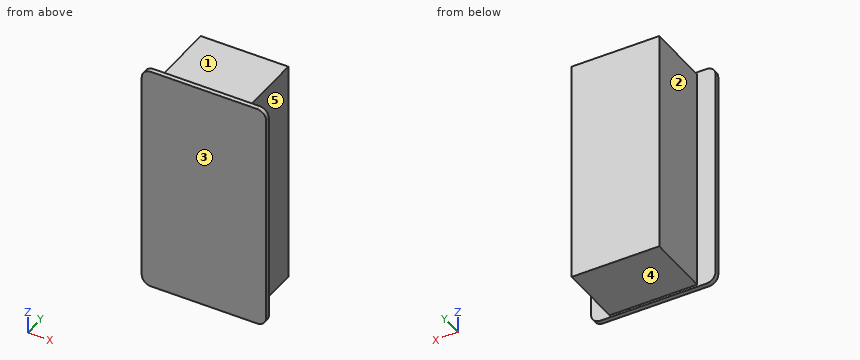
Autodesk Inventor part; units mm, degrees
ref_plane "YZ Plane" through (0, 0, 0) normal (1, 0, 0) x (0, 1, 0)
ref_plane "XZ Plane" through (0, 0, 0) normal (0, 1, 0) x (-1, 0, 0)
ref_plane "XY Plane" through (0, 0, 0) normal (0, 0, 1) x (1, 0, 0)
sketch "Sketch1" plane through (0, 0, 0) normal (0, 1, 0) x (-1, 0, 0)
  line L0 (-13.5, 25) -> (-13.5, -25)
  line L1 (-13.5, -25) -> (13.5, -25)
  line L2 (13.5, -25) -> (13.5, 25)
  line L3 (13.5, 25) -> (-13.5, 25)
  line L4 (-13.5, 25) -> (13.5, -25) construction
  line L5 (-13.5, -25) -> (13.5, 25) construction
  point P0 (0, 0)
  dimension "d0" = 50
  dimension "d1" = 27
extrude "Extrusion1" add sketch "Sketch1" along normal blind 1
fillet "Fillet1" radius 2 4 edges at (13.5, 0.5, 25) (-13.5, 0.5, 25) (-13.5, 0.5, -25) (13.5, 0.5, -25)
sketch "Sketch2" plane through (0, 1, 0) normal (0, 1, 0) x (1, 0, 0)
  line L0 (9.5, -24.5) -> (9.5, 24.5)
  line L1 (9.5, 24.5) -> (-9.5, 24.5)
  line L2 (-9.5, 24.5) -> (-9.5, -24.5)
  line L3 (-9.5, -24.5) -> (9.5, -24.5)
  line L4 (9.5, -24.5) -> (-9.5, 24.5) construction
  line L5 (9.5, 24.5) -> (-9.5, -24.5) construction
  point P0 (0, 0)
  dimension "d5" = 49
  dimension "d6" = 19
extrude "Extrusion2" add sketch "Sketch2" along normal blind 14
sketch "Sketch3" plane through (0, 15, 0) normal (0, 1, 0) x (1, 0, 0)
  point P0 (0, 0)
sketch "Sketch4" plane through (0, 15, 0) normal (0, 1, 0) x (1, 0, 0)
  line L0 (-9.2797, -24.5843) -> (-9.5, 24.5) construction
  line L1 (-9.5, 24.5) -> (9.2797, 24.5843) construction
  line L2 (9.2797, 24.5843) -> (9.5, -24.5) construction
  line L3 (9.5, -24.5) -> (-9.2797, -24.5843) construction
  line L4 (9.5, -24.5) -> (9.5, 24.5)
  line L5 (9.5, 24.5) -> (-9.5, 24.5)
  line L6 (-9.5, 24.5) -> (-9.5, -24.5)
  line L7 (-9.5, -24.5) -> (9.5, -24.5)
  point P0 (0, 0)
decal "Decal1"
properties part number "Digit Display"
Read the model definition and answer for the solid it produces. Units are mm, in the model's axes. Face numbers are marked on the shaded views. A direction names the side the tool comes from. Give positions to 0.01 mm unless a question says otherwise; leave off trailing zeros. Write each loop counter-clockwise with the first axis right and the second up, starting at its lowest first coordinate (ties: lowest second). Pieces come first, ordered by that corner, then holes. Notation, with made-up numbers: (85, -15.75) -> (118, -15.75) arc R26 cw to (118, 5.25) -> close; hole circle Ø1 at (15.25, 34). An arc over 180 degrees is marked (long way). Answer as a JSON object with one key per item and string values. Group by question number.
1) Find section B-B (z = 2.5). Write down the section's boundary in (x, y).
2) Consider L1, parallel to Z at x = 1.25, y = 10; L2, parallel to X at y = 13.5, z = -8; L3, parallel to Y at x = 9.75, z = -16.5. Determine where each line is inside the solid, lowest interval first. Write a range as from..to.
3) A tool of negligible diameter and unlimited length cuts with its end or side. For the marked faces 1, 2, 3, 4 and 5, from which of +Z, -Z, +X, -X, +Y, -Y can it reach the whole face along a straight path? Write none if from no direction.
4) Find section C-C (y = 11). Write down the section's boundary in (x, z).
5) Each of these flat-tipped pins is pushed along its axis until it touches: P1, Ø8, axis at y = 9, z = 8, coming from the +X side; P2, Ø7, axis at x = -2.5, y = 10.5, coming from the +Z side; P3, Ø7, axis at x = 4.5, y = 7.5, coming from the -Z side. Where does it stop, or does it pass through?
6) Find section A-A (x = 8.5). Write down the section's boundary in (y, z), and give its area (3 significant figures).
Values follow:
{
 "1": {"outline": "(-13.5, 0) -> (13.5, 0) -> (13.5, 1) -> (9.5, 1) -> (9.5, 15) -> (-9.5, 15) -> (-9.5, 1) -> (-13.5, 1) -> close"},
 "2": {"L1": "z = -24.5..24.5", "L2": "x = -9.5..9.5", "L3": "y = 0..1"},
 "3": {"face 1": "+Z, +X, -X, +Y", "face 2": "+Z, -Z, -X, +Y", "face 3": "+Z, -Z, +X, -X, -Y", "face 4": "-Z, +X, -X, +Y", "face 5": "+Z, -Z, +X, +Y"},
 "4": {"outline": "(-9.5, -24.5) -> (9.5, -24.5) -> (9.5, 24.5) -> (-9.5, 24.5) -> close"},
 "5": {"P1": "stops at x = 9.5", "P2": "stops at z = 24.5", "P3": "stops at z = -24.5"},
 "6": {"outline": "(0, -25) -> (1, -25) -> (1, -24.5) -> (15, -24.5) -> (15, 24.5) -> (1, 24.5) -> (1, 25) -> (0, 25) -> close", "area": "736 mm2"}
}
